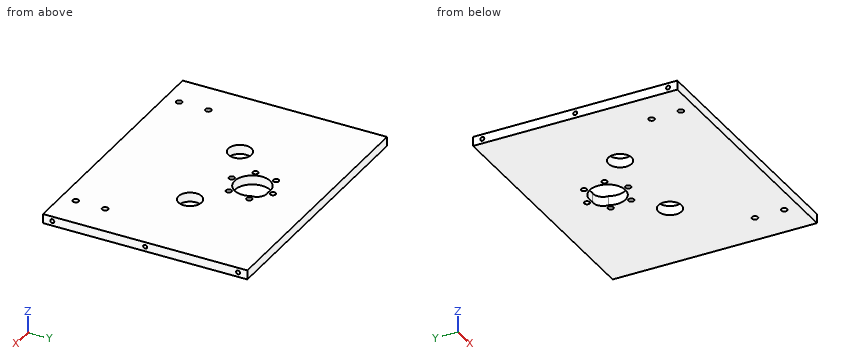
```python
from build123d import *

# Parameters (mm, degrees)
SKETCH1_W                          = 177.8
SKETCH1_H                          = 139.7
BOSS_EXTRUDE1_DEPTH                = 6.35
SKETCH2_R                          = 7.9375
CUT_EXTRUDE1_DEPTH                 = 7.35
TAP_DRILL_FOR_6_32_TAP1_AT_2_COUNT = 2
TAP_DRILL_FOR_6_32_TAP1_AT_2_PITCH = 63.5
TAP_DRILL_FOR_6_32_TAP1_AT_3_COUNT = 2
TAP_DRILL_FOR_6_32_TAP1_AT_3_PITCH = 127
TAP_DRILL_FOR_10_32_TAP1_D         = 4.0386
SKETCH20_R                         = 12.192
CUT_EXTRUDE4_DEPTH                 = 7.35
F_6_CLEARANCE_HOLE1_D              = 3.7973
CIRPATTERN1_COUNT                  = 6
CUT_EXTRUDE5_DEPTH                 = 7.35


with BuildPart() as part:
    # Sketch1 → Boss-Extrude1 (new body)
    with BuildSketch(Plane.XY):
        Rectangle(SKETCH1_W, SKETCH1_H)
    extrude(amount=BOSS_EXTRUDE1_DEPTH)

    # Sketch2 → Cut-Extrude1 (cut, through all)
    with BuildSketch(Plane.XY.offset(6.35)):
        with Locations((-31.75, 0)):
            Circle(SKETCH2_R)
        with Locations((31.75, 0)):
            Circle(SKETCH2_R)
    extrude(amount=-CUT_EXTRUDE1_DEPTH, mode=Mode.SUBTRACT)

    # Sketch17 → Tap Drill for #6-32 Tap1 (revolve, cut)
    with BuildSketch(Plane(origin=(88.9, 63.5, 3.175), x_dir=(0, 0, -1), z_dir=(0, 1, 0))):
        Polygon((0, 0), (0, 13.51269403), (1.35255, 12.7), (1.35255, 0), align=None)
    tap_drill_for_6_32_tap1 = revolve(axis=Axis((95.25, 63.5, 3.175), (-1, 0, 0)), mode=Mode.SUBTRACT)

    # Tap Drill for #6-32 Tap1 at 2: Tap Drill for #6-32 Tap1 ×2
    with Locations(*[(0, -i * TAP_DRILL_FOR_6_32_TAP1_AT_2_PITCH, 0) for i in range(1, TAP_DRILL_FOR_6_32_TAP1_AT_2_COUNT)]):
        add(tap_drill_for_6_32_tap1, mode=Mode.SUBTRACT)

    # Tap Drill for #6-32 Tap1 at 3: Tap Drill for #6-32 Tap1 ×2
    with Locations(*[(0, -i * TAP_DRILL_FOR_6_32_TAP1_AT_3_PITCH, 0) for i in range(1, TAP_DRILL_FOR_6_32_TAP1_AT_3_COUNT)]):
        add(tap_drill_for_6_32_tap1, mode=Mode.SUBTRACT)

    # Mirror2: Tap Drill for #6-32 Tap1 across plane
    add(tap_drill_for_6_32_tap1.mirror(Plane(origin=(0, 0, 0), x_dir=(0, 0, 1), z_dir=(1, 0, 0))), mode=Mode.SUBTRACT)

    # Mirror2 copy 1 sketch → Mirror2 copy 1 (revolve, cut)
    with BuildSketch(Plane(origin=(-88.9, 0, 3.175), x_dir=(0, 0, -1), z_dir=(0, 1, 0))):
        Polygon((0, 0), (0, -13.51269403), (1.35255, -12.7), (1.35255, 0), align=None)
    revolve(axis=Axis((-95.25, 0, 3.175), (-1, 0, 0)), mode=Mode.SUBTRACT)

    # Mirror2 copy 2 sketch → Mirror2 copy 2 (revolve, cut)
    with BuildSketch(Plane(origin=(-88.9, -63.5, 3.175), x_dir=(0, 0, -1), z_dir=(0, 1, 0))):
        Polygon((0, 0), (0, -13.51269403), (1.35255, -12.7), (1.35255, 0), align=None)
    revolve(axis=Axis((-95.25, -63.5, 3.175), (-1, 0, 0)), mode=Mode.SUBTRACT)

    # Tap Drill for #10-32 Tap1 (through all)
    with Locations(Plane.XY.offset(6.35)):
        with Locations((-65.750000072, -59.85), (-65.750000072, -39.85)):
            tap_drill_for_10_32_tap1 = Hole(TAP_DRILL_FOR_10_32_TAP1_D / 2)

    # Mirror3: Tap Drill for #10-32 Tap1 across plane
    add(tap_drill_for_10_32_tap1.mirror(Plane(origin=(0, 0, 0), x_dir=(0, 0, 1), z_dir=(1, 0, 0))), mode=Mode.SUBTRACT)

    # Sketch20 → Cut-Extrude4 (cut, through all)
    with BuildSketch(Plane.XY.offset(6.35)):
        with Locations((0, 25.577056324)):
            Circle(SKETCH20_R)
    extrude(amount=-CUT_EXTRUDE4_DEPTH, mode=Mode.SUBTRACT)

    # #6 Clearance Hole1 (through all)
    with Locations(Plane.XY.offset(6.35)):
        with Locations((2.308510654, 40.904181905)):
            f_6_clearance_hole1 = Hole(F_6_CLEARANCE_HOLE1_D / 2)

    # CirPattern1: #6 Clearance Hole1 ×6 about axis
    cirpattern1_axis = Axis((0, 25.577056324, 0), (0, 0, 1))
    for i in range(1, CIRPATTERN1_COUNT):
        add(f_6_clearance_hole1.rotate(cirpattern1_axis, i * 360 / CIRPATTERN1_COUNT), mode=Mode.SUBTRACT)

    # Sketch23 → Cut-Extrude5 (cut, through all)
    with BuildSketch(Plane(origin=(0, 0, 0), x_dir=(-1, 0, 0), z_dir=(0, 0, -1))):
        with BuildLine():
            ThreePointArc((0.824054314, 35.186643177), (-8.500139633, 36.23824065), (-9.551737105, 26.914046703))
            ThreePointArc((-9.551737105, 26.914046703), (-0.227543158, 25.862449231), (0.824054314, 35.186643177))
        make_face()
    extrude(amount=-CUT_EXTRUDE5_DEPTH, mode=Mode.SUBTRACT)


solid = part.part
```
The model under review builds one solid part; all positions refer to its coordinate system, in mm. Round coordinates to 2 decimals unless told otherwise and drop trailing zeros. Write each loop counter-clockwise with the first axis right and the second up, starting at its lowest first coordinate (ties: lowest second). Pieces come first, ordered by that corner, then holes. Notation, with made-up numbers: (38.25, 54.25) - (63.25, 54.25) arc R23 cw to (63.25, 76.25) - close; hole circle Ø11 at (23.25, 29.5). An arc over 180 degrees is marked (long way). One line per question, with ' | ' between items.
Item 1: Add section A-A, the plane y = -59.85. Give the boundary of the cut face in (x, z), then the cut area to 3 significant figures.
Resolved:
outline: (-88.9, 0) - (-67.77, 0) - (-67.77, 6.35) - (-88.9, 6.35) - close; (-63.73, 0) - (63.73, 0) - (63.73, 6.35) - (-63.73, 6.35) - close; (67.77, 0) - (88.9, 0) - (88.9, 6.35) - (67.77, 6.35) - close | area: 1,080 mm2
Item 2: To check wall thickness, follow probe 1 along X at (y, z) = (3, 5); probe 2 along X at (y, z) = (-0.5, 4); probe 3 along Y at (x, z) = (-33, 4.5). State the ranges of each line that lie inside material, in increasing order.
Resolved:
probe 1: x = -88.9 to -39.1, -24.4 to 24.4, 39.1 to 88.9 | probe 2: x = -75.97 to -39.67, -23.83 to 23.83, 39.67 to 75.97 | probe 3: y = -69.85 to -7.84, 7.84 to 69.85
Item 3: Add section C-C, the plane x = -65.75. Give the boundary of the cut face in (y, z), then the cut area to 3 significant figures.
Resolved:
outline: (-69.85, 0) - (-61.87, 0) - (-61.87, 6.35) - (-69.85, 6.35) - close; (-57.83, 0) - (-41.87, 0) - (-41.87, 6.35) - (-57.83, 6.35) - close; (-37.83, 0) - (69.85, 0) - (69.85, 6.35) - (-37.83, 6.35) - close | area: 836 mm2
Item 4: For P1, Ø1.6, axis at y = 63.5, z = 3.175, coming from the +X side; P2, Ø2.5, axis at x = 65.75, y = -39.85, coming from the -Z side; P3, Ø1.6, axis at y = -63.5, z = 3.175, coming from the -X side, all flat-tipped, find the tip position at first contact; note any pin that passes through.
Resolved:
P1: stops at x = 75.87 | P2: passes through | P3: stops at x = -75.87
Item 5: Add section B-B, the plane x = 31.75. Give the boundary of the cut face in (y, z).
Resolved:
outline: (-69.85, 0) - (-7.94, 0) - (-7.94, 6.35) - (-69.85, 6.35) - close; (7.94, 0) - (69.85, 0) - (69.85, 6.35) - (7.94, 6.35) - close
